from build123d import *

# Parameters (mm, degrees)
SKETCH1_W            = 15.9
SKETCH1_H            = 7.9
MAIN_BODY_DEPTH      = 9.6
MAIN_BODY_TAPER      = 1
SKETCH2_R            = 2.4
POST_DEPTH           = 1.8
POST_LPATTERN1_COUNT = 2
POST_LPATTERN1_PITCH = 8
SHELL1_T             = -1.2
BODY_FILLET_R        = 0.25
POST_CHAMFER_SIZE    = 0.25


with BuildPart() as part:
    # Sketch1 → Main Body (new body)
    with BuildSketch(Plane.XY):
        with Locations((7.95, 3.95)):
            Rectangle(SKETCH1_W, SKETCH1_H)
    extrude(amount=MAIN_BODY_DEPTH, taper=MAIN_BODY_TAPER)

    # Sketch2 → Post (add)
    with BuildSketch(Plane.XY.offset(9.6)):
        with Locations(Location((3.95, 3.95, 0), (0, 0, 180))):
            Circle(SKETCH2_R)
    post = extrude(amount=POST_DEPTH)

    # Post LPattern1: Post ×2
    with Locations(*[(i * POST_LPATTERN1_PITCH, 0, 0) for i in range(1, POST_LPATTERN1_COUNT)]):
        add(post)

    # Shell1
    shell1_openings = [part.faces().sort_by_distance(p)[0] for p in [
        (7.95, 3.95, 0),
    ]]
    offset(amount=SHELL1_T, openings=shell1_openings, kind=Kind.INTERSECTION)

    # Body Fillet
    body_fillet_edges = [part.edges().sort_by_distance(p)[0] for p in [
        (15.732431377, 3.95, 9.6),
        (6.35, 3.95, 9.6),
        (7.95, 7.732431377, 9.6),
        (14.35, 3.95, 9.6),
        (0.167568623, 3.95, 9.6),
        (0.083784312, 7.816215688, 4.8),
        (15.816215688, 7.816215688, 4.8),
        (15.816215688, 0.083784312, 4.8),
        (0.083784312, 0.083784312, 4.8),
        (7.95, 0.167568623, 9.6),
    ]]
    fillet(body_fillet_edges, radius=BODY_FILLET_R)

    # Post Chamfer
    post_chamfer_edges = [part.edges().sort_by_distance(p)[0] for p in [
        (6.35, 3.95, 11.4),
        (14.35, 3.95, 11.4),
    ]]
    chamfer(post_chamfer_edges, length=POST_CHAMFER_SIZE)


solid = part.part
Check sheet for the modelled part. Datum: model origin and axes. Units: mm. A direction names the side the tool comes from. Give positions to 0.01 mm unless a question says otherwise; leave off trailing zeros. Loops run counter-clockwise (first coordinate to the right, second up) from the corner with the lowest first, then second, coordinate; pieces in that order, holes last. Notation, with made-up numbers: M 28,5 L 43,5 A18 ccw 43,26 Z; hole C -38,-10 d6. An arc over 180 degrees is marked long. Answer as a JSON object with one key per item and string values. Group by question number.
Q1. Cross-section at C-C on y = 1. Record the cut outline in (x, z), then the cut area to 3 significant figures.
Q2. Cross-section at A-A on z = 10.5. Record the cut outline in (x, y), then the cut area to 3 significant figures.
Q3. Access from +Z, -Z, +X, -X, +Y, -Y to the whole of each face (thin tool, end or side, straight path). Record for faces 5 (the flat face through (12, 4, 10.2)), 6 (the flat face through (12, 4, 11.4)).
Q4. Cross-section at B-B on x = 3.95. Record the cut outline in (y, z).
Q5. Release check for a two-part mould opening along Y. For faces 1 (the cylindrical face through (10.805, 3.59, 9.287)), 2 (the flat face through (8, 4, 9.6)), 3 (the cylindrical face through (4.9, 4.68, 9.29)), 4 (the cylindrical face through (10.7, 1.9, 10.5)) record: released by +Y, released by -Y, zero draft, split by the parting line, or undercut.
Q6. Cross-section at D-D on x = 9. Record the cut outline in (y, z), then the cut area to 3 significant figures.
Q7. Material ranges on line 1 along Y through (x, z) = (3.95, 9.35); line 2 along Z through (x, y) = (3, 4.75); line 3 along X through (y, z) = (4.75, 7.75), recorded low to high. Write a range as [from, to].
Q8. Go/stop test with flat-tipped pins: P1, Ø2.5, axis at x = 12, y = 4, coming from the -Z side; P2, Ø3, axis at y = 6, z = 3, coming from the -X side; P3, Ø5, axis at x = 5, z = 3, coming from the -Y side. Record where each tip stops, or that it passes through.
Evaluation:
{
 "1": {"outline": "M 0,0 L 15.9,0 L 15.74,9.35 A0.25 ccw 15.49,9.6 L 0.41,9.6 A0.25 ccw 0.16,9.35 Z", "area": "151 mm2"},
 "2": {"outline": "C 3.95,3.95 d4.8; C 11.95,3.95 d4.8", "area": "36.2 mm2"},
 "3": {"face 5": "-Z", "face 6": "+Z, +X, -X, +Y, -Y"},
 "4": {"outline": "M 0,0 L 1.2,0 L 1.35,8.4 L 2.75,8.4 L 2.75,10.2 L 5.15,10.2 L 5.15,8.4 L 6.55,8.4 L 6.7,0 L 7.9,0 L 7.74,9.35 A0.25 ccw 7.49,9.6 L 6.6,9.6 A0.25 cw 6.35,9.85 L 6.35,11.15 L 6.1,11.4 L 1.8,11.4 L 1.55,11.15 L 1.55,9.85 A0.25 cw 1.3,9.6 L 0.41,9.6 A0.25 ccw 0.16,9.35 Z"},
 "5": {"face 1": "undercut", "face 2": "zero draft", "face 3": "undercut", "face 4": "split by the parting line"},
 "6": {"outline": "M 0,0 L 1.2,0 L 1.35,8.4 L 6.55,8.4 L 6.7,0 L 7.9,0 L 7.74,9.35 A0.25 ccw 7.49,9.6 L 0.41,9.6 A0.25 ccw 0.16,9.35 Z", "area": "29.2 mm2"},
 "7": {"line 1": "y = [0.16, 2.75], [5.15, 7.74]", "line 2": "z = [8.4, 11.4]", "line 3": "x = [0.14, 1.34], [14.56, 15.76]"},
 "8": {"P1": "stops at z = 8.4", "P2": "stops at x = 0.03", "P3": "stops at y = 0.01"}
}
